```python
from build123d import *

# Parameters (mm, degrees)
FASE1_SIZE = 0.8


with BuildPart() as part:
    # Skizze1 → Rotation1 (revolve)
    with BuildSketch(Plane.XY, mode=Mode.PRIVATE) as rotation1_sk:
        Polygon((-2, 24), (-25, 24), (-25, 19), (5, 19), (5, 27), (0, 27), (0, 25.369078951), (0, 23.8), (-2, 23.8), align=None)
    revolve(rotation1_sk.sketch.rotate(Axis((6.5, 0, 0), (-1, 0, 0)), 90), axis=Axis((6.5, 0, 0), (-1, 0, 0)))

    # Fase1
    fase1_edges = [part.edges().sort_by_distance(p)[0] for p in [
        (-25, 0, 24),
        (-25, 0, 19),
        (5, 0, 19),
    ]]
    chamfer(fase1_edges, length=FASE1_SIZE)


solid = part.part
```
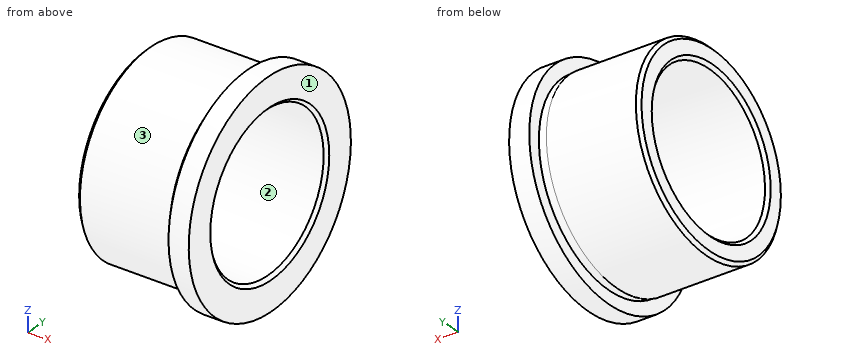
Design review of the part built by this model. Coordinates are the model's own, in mm. Face numbers are marked on the shaded views. Coordinates: 2 decimals unless noted, no trailing zeros. Order: outer loops, then holes, each group sorted by start corner. A loop starts at its lowest first (then second) coordinate and runs counter-clockwise, first axis right, second up.
1) Take a section at A-A, the plane y = 0. Give the boundary of the cut face in (x, z), and give its area (3 significant figures).
2) Mouldability with a two-part tool opening along Y and no side actions: class the marked faces 1, 2 and 3 as +Y half, -Y half, draft (parallel to the pull), parting line (faces both ways), or undercut.
3) Clearance check with flat-ended pins moving along their axes: pin 1 (5 mm diameter, centred on x = -8, y = 0, fed in from -Z); pin 2 (10 mm diameter, centred on x = -18.5, z = 13, fed in from -Y); pin 3 (10 mm diameter, centred on x = -14.5, y = 6, fed in from +Z). State where each tip first meets the part, or that it passes through.
4) Take a section at C-C, the plane x = -19.25. Give the boundary of the cut face in (y, z), and give its area (3 significant figures).
5) Wall thickness on line 1 along Y through (x, z) = (-14.75, 0); line 2 along Y through (x, z) = (-10.5, 10); line 3 along Z through (x, y) = (-18.5, -15) (3 decimals): over which ranges is each line inside the solid? List them lowest first.
Returned:
1. outline: (-25, -23.2) - (-24.2, -24) - (-2, -24) - (-2, -23.8) - (0, -23.8) - (0, -27) - (5, -27) - (5, -19.8) - (4.2, -19) - (-24.2, -19) - (-25, -19.8) - close; (-25, 19.8) - (-24.2, 19) - (4.2, 19) - (5, 19.8) - (5, 27) - (0, 27) - (0, 23.8) - (-2, 23.8) - (-2, 24) - (-24.2, 24) - (-25, 23.2) - close
1. area: 327 mm2
2. face 1: draft
2. face 2: undercut
2. face 3: parting line
3. pin 1: stops at z = -24
3. pin 2: stops at y = -22.63
3. pin 3: stops at z = 23.98
4. outline: circle Ø48 at (0, 0); hole circle Ø38 at (0, 0)
4. area: 675 mm2
5. line 1: y = -24 to -19, 19 to 24
5. line 2: y = -21.82 to -16.16, 16.16 to 21.82
5. line 3: z = -18.735 to -11.662, 11.662 to 18.735
